```python
from build123d import *

# Parameters (mm, degrees)
F1_DEPTH = 101.6
F2_DEPTH = 76.2


with BuildPart() as f1:
    # F0 (on Front) → F1 (new body)
    with BuildSketch(Plane.XZ):
        Polygon((-38.1, 14.664697), (-50.8, 7.332348), (-50.8, 0), (-50.8, -7.332348), (-38.1, -14.664697), (-38.1, -29.329394), (-25.4, -36.661742), (-12.7, -29.329394), (0, -36.661742), (12.7, -29.329394), (25.4, -36.661742), (38.1, -29.329394), (38.1, -14.664697), (50.8, -7.332348), (50.8, 0), (50.8, 7.332348), (38.1, 14.664697), (25.4, 7.332348), (12.7, 14.664697), (0, 7.332348), (-12.7, 14.664697), (-25.4, 7.332348), align=None)
        Polygon((-15.08125, -27.954578), (-25.4, -33.912111), (-35.71875, -27.954578), (-35.71875, -16.039512), (-25.4, -10.081979), (-15.08125, -16.039512), align=None, mode=Mode.SUBTRACT)
        Polygon((-10.31875, -16.039512), (0, -10.081979), (10.31875, -16.039512), (10.31875, -27.954578), (0, -33.912111), (-10.31875, -27.954578), align=None, mode=Mode.SUBTRACT)
        Polygon((-48.41875, 0), (-48.41875, 5.957533), (-38.1, 11.915066), (-27.78125, 5.957533), (-27.78125, 0), (-27.78125, -5.957533), (-38.1, -11.915066), (-48.41875, -5.957533), align=None, mode=Mode.SUBTRACT)
        Polygon((25.4, -10.081979), (35.71875, -16.039512), (35.71875, -27.954578), (25.4, -33.912111), (15.08125, -27.954578), (15.08125, -16.039512), align=None, mode=Mode.SUBTRACT)
        Polygon((48.41875, 0), (48.41875, -5.957533), (38.1, -11.915066), (27.78125, -5.957533), (27.78125, 0), (27.78125, 5.957533), (38.1, 11.915066), (48.41875, 5.957533), align=None, mode=Mode.SUBTRACT)
        Polygon((-12.7, 11.915066), (-2.38125, 5.957533), (-2.38125, 0), (-2.38125, -5.957533), (-12.7, -11.915066), (-23.01875, -5.957533), (-23.01875, 0), (-23.01875, 5.957533), align=None, mode=Mode.SUBTRACT)
        Polygon((23.01875, 5.957533), (23.01875, 0), (23.01875, -5.957533), (12.7, -11.915066), (2.38125, -5.957533), (2.38125, 0), (2.38125, 5.957533), (12.7, 11.915066), align=None, mode=Mode.SUBTRACT)
    extrude(amount=F1_DEPTH)

    # F0 (on Front) → F2 (join)
    with BuildSketch(Plane.XZ):
        Polygon((-38.1, 29.329394), (-38.1, 14.664697), (-25.4, 7.332348), (-12.7, 14.664697), (-12.7, 29.329394), (-25.4, 36.661742), align=None)
        Polygon((-15.08125, 27.954578), (-15.08125, 16.039512), (-25.4, 10.081979), (-35.71875, 16.039512), (-35.71875, 27.954578), (-25.4, 33.912111), align=None, mode=Mode.SUBTRACT)
        Polygon((-12.7, 29.329394), (-12.7, 14.664697), (0, 7.332348), (12.7, 14.664697), (12.7, 29.329394), (0, 36.661742), align=None)
        Polygon((-10.31875, 16.039512), (-10.31875, 27.954578), (0, 33.912111), (10.31875, 27.954578), (10.31875, 16.039512), (0, 10.081979), align=None, mode=Mode.SUBTRACT)
        Polygon((12.7, 29.329394), (12.7, 14.664697), (25.4, 7.332348), (38.1, 14.664697), (38.1, 29.329394), (25.4, 36.661742), align=None)
        Polygon((15.08125, 16.039512), (15.08125, 27.954578), (25.4, 33.912111), (35.71875, 27.954578), (35.71875, 16.039512), (25.4, 10.081979), align=None, mode=Mode.SUBTRACT)
    extrude(amount=F2_DEPTH)


solid = f1.part
```
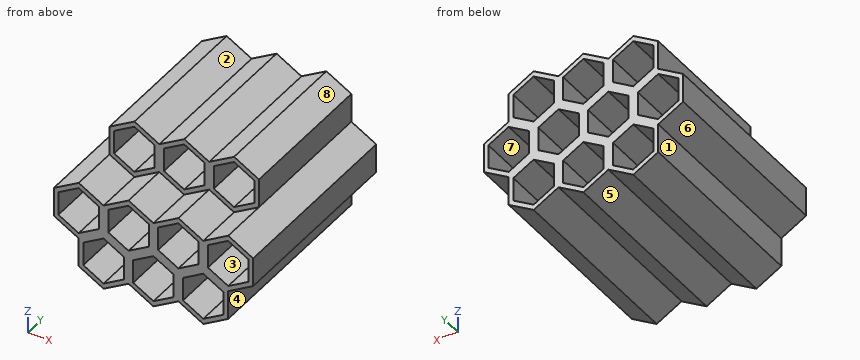
Source: CAD feature listing. Evaluate the final solid. Frame: model axes, mm. Face numbers are marked on the shaded views. A direction names the side the tool comes from. Coordinates: 2 decimals unless noted, no trailing zeros. Order: outer loops, then holes, each group sorted by start corner. A loop starts at its lowest first (then second) coordinate and runs counter-clockwise, first axis right, second up. Notation, with made-up numbers: M -22.5,-24.5 L 23.5,-24.5 A26 cw 23.5,3.5 Z; hole C -0.5,39.5 d11. An arc over 180 degrees is marked long. Write each question's results on one line, items separated by ' | '. Start each with the question number.
1) Access query for the marked faces 1, 2, 3 and 4. Directions: +Z, -Z, +X, -X, +Y, -Y. A direction counts if a zero-diameter tool reaches every point of the face in a straight line with its end or side. Return the directions, or none.
2) Contact query for flat-ended pins moving along their axis: pin 1 Ø16 at (y, z) = (-31.5, 21) entering from -X; pin 2 Ø13 at (y, z) = (-56, -22) entering from +X; pin 3 Ø9.5 at (y, z) = (-35.5, -20) entering from -X. Output: stop coordinate, or through.
3) Draft query along X for the marked faces 5, 6, 7 and 8. Return one class per face: released by +X, released by -X, zero draft, split by the parting line, or undercut.
4) Section query B-B (x = 40). Return the cut outline in (y, z), plus the area to 3 significant figures.
5) Line query: line 1 (X direction, y = -66.5, z = -18); line 2 (X direction, y = -25, z = 3.5); line 3 (X direction, y = -16.5, z = 32.5). Output: solid intervals per line, ascending. Write a range as from..to.
6) Section query A-A (z = -18). Return the cut outline in (x, y).
7) Section query C-C (z = -32). Return the cut outline in (x, y).
8) Section query D-D (y = -14.5). Give the number of separate pieces and of enclosed holes in the cut face, plus the area to 3 significant figures.
Answers:
1) face 1: -Z, -X, +Y, -Y | face 2: +Z, +Y, -Y | face 3: +Y, -Y | face 4: -Z, +X, +Y, -Y
2) pin 1: stops at x = -40.98 | pin 2: stops at x = 38.1 | pin 3: stops at x = -38.1
3) face 5: undercut | face 6: released by -X | face 7: undercut | face 8: released by +X
4) outline: M -101.6,-13.57 L 0,-13.57 L 0,-10.82 L -101.6,-10.82 Z; M -101.6,10.82 L 0,10.82 L 0,13.57 L -101.6,13.57 Z | area: 559 mm^2
5) line 1: x = -38.1..-35.72, -15.08..-10.32, 10.32..15.08, 35.72..38.1 | line 2: x = -50.8..-48.42, -27.78..-23.02, -2.38..2.38, 23.02..27.78, 48.42..50.8 | line 3: x = -32.61..-27.85, -22.95..-18.19, -7.21..-2.45, 2.45..7.21, 18.19..22.95, 27.85..32.61
6) outline: M -38.1,-101.6 L -35.72,-101.6 L -35.72,0 L -38.1,0 Z; M -15.08,-101.6 L -10.32,-101.6 L -10.32,0 L -15.08,0 Z; M 10.32,-101.6 L 15.08,-101.6 L 15.08,0 L 10.32,0 Z; M 35.72,-101.6 L 38.1,-101.6 L 38.1,0 L 35.72,0 Z
7) outline: M -33.47,-101.6 L -28.71,-101.6 L -28.71,0 L -33.47,0 Z; M -22.09,-101.6 L -17.33,-101.6 L -17.33,0 L -22.09,0 Z; M -8.07,-101.6 L -3.31,-101.6 L -3.31,0 L -8.07,0 Z; M 3.31,-101.6 L 8.07,-101.6 L 8.07,0 L 3.31,0 Z; M 17.33,-101.6 L 22.09,-101.6 L 22.09,0 L 17.33,0 Z; M 28.71,-101.6 L 33.47,-101.6 L 33.47,0 L 28.71,0 Z
8) separate pieces: 1 | enclosed holes: 10 | area: 1,900 mm^2
